Check sheet for the modelled part. Datum: model origin and axes. Units: mm. A direction names the side the tool comes from. Round coordinates to 2 decimals unless told otherwise and drop trailing zeros. Loops run counter-clockwise (first coordinate to the right, second up) from the corner with the lowest first, then second, coordinate; pieces in that order, holes last. Notation, with made-up numbers: (75.25, -26) - (114.25, -26) arc R21 cw to (114.25, 7) - close; hole circle Ø2 at (2, -11.5). An arc over 180 degrees is marked (long way). Put each result on its own line as item: value.
```python
from build123d import *

# Parameters (mm, degrees)
F0_R          = 22.225
F1_DEPTH      = 6.35
F2_SIZE       = 1.905
F4_DEPTH      = 50.8
F8_DEPTH      = 25.4
F8_DEPTH_BACK = 25.4
F9_SIZE       = 5.08
F10_SIZE      = 5.08


with BuildPart() as f1:
    # F0 (on Top) → F1 (new body)
    with BuildSketch(Plane.XY):
        with BuildLine():
            ThreePointArc((-76.2, 0), (0, -76.2), (76.2, 0))
            ThreePointArc((76.2, 0), (0, 76.2), (-76.2, 0))
        make_face()
        with BuildLine():
            ThreePointArc((-36.3505191374, -55.3531540115), (-40.5694607495, -55.5302656455), (-41.2330473061, -51.3600750337))
            Line((-41.2330473061, -51.3600750337), (-20.5013866713, -22.8161053906))
            ThreePointArc((-20.5013866713, -22.8161053906), (-16.2954133846, -21.961508124), (-15.0808678012, -26.0779904576))
            Line((-15.0808678012, -26.0779904576), (-36.3505191374, -55.3531540115))
        make_face(mode=Mode.SUBTRACT)
        with BuildLine():
            ThreePointArc((3.1275798593, -66.1479413497), (-0.1815119967, -68.7710593314), (-3.1695413391, -65.7873506482))
            Line((-3.1695413391, -65.7873506482), (-3.174999962, -30.5090297434))
            ThreePointArc((-3.174999962, -30.5090297434), (-0.2746157651, -27.3454369619), (3.1275798593, -29.9618491446))
            Line((3.1275798593, -29.9618491446), (3.1275798593, -66.1479413497))
        make_face(mode=Mode.SUBTRACT)
        with BuildLine():
            ThreePointArc((-61.9439553323, -23.4153432254), (-65.4612544013, -21.0787978873), (-63.546930662, -17.314996421))
            Line((-63.546930662, -17.314996421), (-29.9969404887, -6.4082042695))
            ThreePointArc((-29.9969404887, -6.4082042695), (-26.0919169519, -8.189029627), (-27.5289365415, -12.233225774))
            Line((-27.5289365415, -12.233225774), (-61.9439553323, -23.4153432254))
        make_face(mode=Mode.SUBTRACT)
        with BuildLine():
            ThreePointArc((41.4110496523, -51.6764633782), (40.2757681695, -55.743645795), (36.1046216907, -55.086094345))
            Line((36.1046216907, -55.086094345), (15.3641288185, -26.548541698))
            ThreePointArc((15.3641288185, -26.548541698), (15.8510757428, -22.2843383176), (20.1413983161, -22.4012998243))
            Line((20.1413983161, -22.4012998243), (41.4110496523, -51.6764633782))
        make_face(mode=Mode.SUBTRACT)
        with BuildLine():
            ThreePointArc((63.8769059879, -17.4663328146), (65.349073818, -21.4240542218), (61.5880463856, -23.3438223094))
            Line((61.5880463856, -23.3438223094), (28.0346825979, -12.4474130757))
            ThreePointArc((28.0346825979, -12.4474130757), (25.9221950752, -8.7113798527), (29.4618871971, -6.2842153632))
            Line((29.4618871971, -6.2842153632), (63.8769059879, -17.4663328146))
        make_face(mode=Mode.SUBTRACT)
        Polygon((-58.42, -7.62), (-58.42, 0), (-58.42, 7.62), (-50.038, 7.62), (-50.038, -7.62), align=None, mode=Mode.SUBTRACT)
        with BuildLine():
            ThreePointArc((-63.8769059879, 17.4663328146), (-65.349073818, 21.4240542218), (-61.5880463856, 23.3438223094))
            Line((-61.5880463856, 23.3438223094), (-28.0346825979, 12.4474130757))
            ThreePointArc((-28.0346825979, 12.4474130757), (-25.9221950752, 8.7113798527), (-29.4618871971, 6.2842153632))
            Line((-29.4618871971, 6.2842153632), (-63.8769059879, 17.4663328146))
        make_face(mode=Mode.SUBTRACT)
        with BuildLine():
            ThreePointArc((-41.4110496523, 51.6764633782), (-40.2757681695, 55.743645795), (-36.1046216907, 55.086094345))
            Line((-36.1046216907, 55.086094345), (-15.3641288185, 26.548541698))
            ThreePointArc((-15.3641288185, 26.548541698), (-15.8510757428, 22.2843383176), (-20.1413983161, 22.4012998243))
            Line((-20.1413983161, 22.4012998243), (-41.4110496523, 51.6764633782))
        make_face(mode=Mode.SUBTRACT)
        Circle(F0_R, mode=Mode.SUBTRACT)
        Polygon((58.42, 7.62), (58.42, 0), (58.42, -7.62), (50.038, -7.62), (50.038, 7.62), align=None, mode=Mode.SUBTRACT)
        with BuildLine():
            ThreePointArc((61.9439553323, 23.4153432254), (65.4612544013, 21.0787978873), (63.546930662, 17.314996421))
            Line((63.546930662, 17.314996421), (29.9969404887, 6.4082042695))
            ThreePointArc((29.9969404887, 6.4082042695), (26.0919169519, 8.189029627), (27.5289365415, 12.233225774))
            Line((27.5289365415, 12.233225774), (61.9439553323, 23.4153432254))
        make_face(mode=Mode.SUBTRACT)
        with BuildLine():
            ThreePointArc((3.174999962, 30.5090297434), (0.2746157651, 27.3454369619), (-3.1275798593, 29.9618491446))
            Line((-3.1275798593, 29.9618491446), (-3.1275798593, 66.1479413497))
            ThreePointArc((-3.1275798593, 66.1479413497), (0.1815119967, 68.7710593314), (3.1695413391, 65.7873506482))
            Line((3.1695413391, 65.7873506482), (3.174999962, 30.5090297434))
        make_face(mode=Mode.SUBTRACT)
        with BuildLine():
            ThreePointArc((36.3505191374, 55.3531540115), (40.5694607495, 55.5302656455), (41.2330473061, 51.3600750337))
            Line((41.2330473061, 51.3600750337), (20.5013866713, 22.8161053906))
            ThreePointArc((20.5013866713, 22.8161053906), (16.2954133846, 21.961508124), (15.0808678012, 26.0779904576))
            Line((15.0808678012, 26.0779904576), (36.3505191374, 55.3531540115))
        make_face(mode=Mode.SUBTRACT)
    extrude(amount=F1_DEPTH)

    # F2
    f2_edges = [f1.edges().sort_by_distance(p)[0] for p in [
        (58.42, 7.62, 3.175),
        (50.038, 7.62, 3.175),
        (58.42, -7.62, 3.175),
        (50.038, -7.62, 3.175),
        (-50.038, 7.62, 3.175),
        (-58.42, 7.62, 3.175),
        (-50.038, -7.62, 3.175),
        (-58.42, -7.62, 3.175),
    ]]
    chamfer(f2_edges, length=F2_SIZE)

    # F3 (on face) → F4 (join)
    with BuildSketch(Plane(origin=(0, 0, 0), x_dir=(1, 0, 0), z_dir=(0, 0, -1))):
        with BuildLine():
            ThreePointArc((-36.407482317, 44.0524429667), (-40.3640168655, 45.6764662753), (-44.310067169, 44.0271317603))
            Line((-44.310067169, 44.0271317603), (-40.5403775713, 40.2815129604))
            ThreePointArc((-40.5403775713, 40.2815129604), (-38.5201020718, 42.2175820764), (-36.407482317, 44.0524429667))
        make_face()
        with BuildLine():
            Line((-40.5403775713, 40.2815129604), (-36.3821711106, 36.1498581148))
            ThreePointArc((-36.3821711106, 36.1498581148), (-35.1800623463, 37.9583303415), (-34.7581191398, 40.0884949375))
            ThreePointArc((-34.7581191398, 40.0884949375), (-35.1869115182, 42.2351948973), (-36.407482317, 44.0524429667))
            ThreePointArc((-36.407482317, 44.0524429667), (-38.5201020718, 42.2175820764), (-40.5403775713, 40.2815129604))
        make_face()
        with BuildLine():
            Line((40.4111525448, -40.4111525448), (36.4618960058, -36.4618960058))
            ThreePointArc((36.4618960058, -36.4618960058), (34.9572040364, -40.2442749258), (36.4178321079, -44.0438872554))
            ThreePointArc((36.4178321079, -44.0438872554), (38.457410353, -42.2746979757), (40.4111525448, -40.4111525448))
        make_face()
        with BuildLine():
            ThreePointArc((36.4178321079, -44.0438872554), (40.3228976199, -45.8603299081), (44.359963556, -44.359963556))
            Line((44.359963556, -44.359963556), (40.4111525448, -40.4111525448))
            ThreePointArc((40.4111525448, -40.4111525448), (38.457410353, -42.2746979757), (36.4178321079, -44.0438872554))
        make_face()
        with BuildLine():
            ThreePointArc((-44.2847559626, 36.1245469084), (-40.3282214141, 34.5005235998), (-36.3821711106, 36.1498581148))
            Line((-36.3821711106, 36.1498581148), (-40.5403775713, 40.2815129604))
            ThreePointArc((-40.5403775713, 40.2815129604), (-42.4634656081, 38.248876958), (-44.2847559626, 36.1245469084))
        make_face()
        with BuildLine():
            Line((-40.5403775713, 40.2815129604), (-44.310067169, 44.0271317603))
            ThreePointArc((-44.310067169, 44.0271317603), (-45.9340904775, 40.0705972119), (-44.2847559626, 36.1245469084))
            ThreePointArc((-44.2847559626, 36.1245469084), (-42.4634656081, 38.248876958), (-40.5403775713, 40.2815129604))
        make_face()
        with BuildLine():
            ThreePointArc((46.1331096706, -40.2767498912), (45.6501506831, -38.004240208), (44.2847559626, -36.1245469084))
            ThreePointArc((44.2847559626, -36.1245469084), (42.4021576862, -38.3168308131), (40.4111525448, -40.4111525448))
            Line((40.4111525448, -40.4111525448), (44.359963556, -44.359963556))
            ThreePointArc((44.359963556, -44.359963556), (45.6706900042, -42.5025464327), (46.1331096706, -40.2767498912))
        make_face()
        with BuildLine():
            ThreePointArc((40.4111525448, -40.4111525448), (42.4021576862, -38.3168308131), (44.2847559626, -36.1245469084))
            ThreePointArc((44.2847559626, -36.1245469084), (40.3043593055, -34.6939384792), (36.4618960058, -36.4618960058))
            Line((36.4618960058, -36.4618960058), (40.4111525448, -40.4111525448))
        make_face()
    extrude(amount=F4_DEPTH)

    # F7 (on face) → F8 (cut, two sides)
    with BuildSketch(Plane(origin=(0, 0, 0), x_dir=(-0.7071067812, -0.7071067812, 0), z_dir=(-0.7071067812, 0.7071067812, 0))) as f8_sk:
        Polygon((62.0108805597, -54.0438257158), (62.0108805597, -52.6354536414), (56.3773885369, -43.801125139), (51.3840802014, -54.0438257158), align=None)
        Polygon((-51.3840802014, -54.0438257158), (-56.3773885369, -43.801125139), (-62.0108805597, -52.6354536414), (-62.0108805597, -54.0438257158), align=None)
    extrude(amount=-F8_DEPTH, mode=Mode.SUBTRACT)
    extrude(f8_sk.sketch, amount=F8_DEPTH_BACK, mode=Mode.SUBTRACT)

    # F9
    f9_edges = [f1.edges().sort_by_distance(p)[0] for p in [
        (-76.2, 0, 0),
    ]]
    chamfer(f9_edges, length=F9_SIZE)

    # F10
    f10_edges = [f1.edges().sort_by_distance(p)[0] for p in [
        (-22.225, 0, 0),
    ]]
    chamfer(f10_edges, length=F10_SIZE)


solid = f1.part
```
Item 1: Section check C-C on y = 0. Enter the section's corners in (x, z) (3 decimals).
Filled sheet:
outline: (-76.2, 5.08) - (-71.12, 0) - (-58.42, 0) - (-58.42, 6.35) - (-76.2, 6.35) - close; (-50.038, 0) - (-27.305, 0) - (-22.225, 5.08) - (-22.225, 6.35) - (-50.038, 6.35) - close; (22.225, 5.08) - (27.305, 0) - (50.038, 0) - (50.038, 6.35) - (22.225, 6.35) - close; (58.42, 0) - (71.12, 0) - (76.2, 5.08) - (76.2, 6.35) - (58.42, 6.35) - close
Item 2: Section check A-A on x = 0. Enter the section's corners in (y, z) (3 decimals).
Filled sheet:
outline: (-76.2, 5.08) - (-71.12, 0) - (-68.776, 0) - (-68.776, 6.35) - (-76.2, 6.35) - close; (-27.334, 0) - (-27.305, 0) - (-22.225, 5.08) - (-22.225, 6.35) - (-27.334, 6.35) - close; (22.225, 5.08) - (27.305, 0) - (27.334, 0) - (27.334, 6.35) - (22.225, 6.35) - close; (68.776, 0) - (71.12, 0) - (76.2, 5.08) - (76.2, 6.35) - (68.776, 6.35) - close
Item 3: Tool access check on faces 1 (the conical face through (-4.87, -21.94, 4.83)), 2 (the flat face through (-31.012, -37.288, 3.131)). Record the directions out of +Z, -Z, +X, -X, +Y, -Y that give a thin tool (end or side, any length) a straight path to the whole face; none if there is none.
Filled sheet:
face 1: -Z
face 2: +Z, -Z
Item 4: Go/stop test with flat-tipped pins: pin 1 (5 mm diameter, centred on y = 56, z = 2, fed in from +X); pin 2 (1.9 mm diameter, centred on y = 2.5, z = 3, fed in from -X); pin 3 (2.5 mm diameter, centred on x = 55, z = 3, fed in from -Y). Record where each tip stops, or that it passes through.
Filled sheet:
pin 1: x = 51.7
pin 2: x = -75.03
pin 3: y = -51.96
Item 5: Thickness scan on line 1 (Y direction, x = 0, z = 6) (3 decimals); line 2 (Y direction, x = 0, z = 5) (3 decimals); line 3 (X direction, y = 0, z = 5) (3 decimals). Record the ranges inside material, lowest first. Write a range as from..to.
Filled sheet:
line 1: -76.2..-68.776, -27.334..-22.225, 22.225..27.334, 68.776..76.2
line 2: -76.12..-68.776, -27.334..-22.305, 22.305..27.334, 68.776..76.12
line 3: -76.12..-58.42, -50.038..-22.305, 22.305..50.038, 58.42..76.12
Item 6: Section check B-B on z = -9. Enter the section's corners in (x, y), then the cut area to 3 significant figures.
Filled sheet:
outline: circle Ø11.18 at (-40.35, -40.09); circle Ø11.18 at (40.55, 40.28)
area: 196 mm²
